from build123d import *

# Parameters (mm, degrees)
SKETCH1_W           = 12.5
SKETCH1_H           = 14
BOSS_EXTRUDE1_DEPTH = 5
CUT_EXTRUDE1_START  = -4.5
SKETCH3_W           = 0.63999998
SKETCH3_H           = 0.639999981
SKETCH3_W_2         = 0.639999981
CUT_EXTRUDE1_DEPTH  = 4.5
CHAMFER1_SIZE       = 0.5
CHAMFER1_SIZE2      = 0.181985117
SKETCH4_W           = 1.639999981
SKETCH4_H           = 1.639999981
SKETCH4_W_2         = 1.63999998
CUT_EXTRUDE2_DEPTH  = 6


with BuildPart() as part:
    # Sketch1 → Boss-Extrude1 (new body)
    with BuildSketch(Plane(origin=(0, 0, 0), x_dir=(1, 0, 0), z_dir=(0, 1, 0))):
        Rectangle(SKETCH1_W, SKETCH1_H)
    extrude(amount=BOSS_EXTRUDE1_DEPTH)

    # Sketch3 → Cut-Extrude1 (cut)
    with BuildSketch(Plane.XY.offset(7).offset(CUT_EXTRUDE1_START)):
        with Locations((-5.080001681, 1.230026097)):
            Rectangle(SKETCH3_W, SKETCH3_H)
        with Locations((-2.540001758, 1.230026097)):
            Rectangle(SKETCH3_W_2, SKETCH3_H)
        with Locations((-1.834e-06, 1.230026097)):
            Rectangle(SKETCH3_W_2, SKETCH3_H)
        with Locations((2.539998088, 1.230026097)):
            Rectangle(SKETCH3_W_2, SKETCH3_H)
        with Locations((5.079998012, 1.230026097)):
            Rectangle(SKETCH3_W_2, SKETCH3_H)
        with Locations((5.079998012, 3.770026019)):
            Rectangle(SKETCH3_W_2, SKETCH3_H)
        with Locations((2.539998088, 3.770026019)):
            Rectangle(SKETCH3_W_2, SKETCH3_H)
        with Locations((-1.834e-06, 3.770026019)):
            Rectangle(SKETCH3_W_2, SKETCH3_H)
        with Locations((-2.540001758, 3.770026019)):
            Rectangle(SKETCH3_W_2, SKETCH3_H)
        with Locations((-5.080001681, 3.770026019)):
            Rectangle(SKETCH3_W, SKETCH3_H)
    extrude(amount=CUT_EXTRUDE1_DEPTH, mode=Mode.SUBTRACT)

    # Chamfer1
    chamfer1_edges = [part.edges().sort_by_distance(p)[0] for p in [
        (4.759998021, 1.230026096, 7),
        (5.079998011, 0.910026106, 7),
        (2.539998088, 1.550026087, 7),
        (2.219998098, 1.230026096, 7),
        (2.539998088, 0.910026106, 7),
        (2.859998079, 1.230026096, 7),
        (0.319998156, 1.230026096, 7),
        (-1.835e-06, 1.550026087, 7),
        (-0.320001825, 1.230026096, 7),
        (-1.835e-06, 0.910026106, 7),
        (-2.220001767, 1.230026096, 7),
        (-2.540001758, 1.550026087, 7),
        (-2.860001748, 1.230026096, 7),
        (-2.540001758, 0.910026106, 7),
        (-5.080001681, 0.910026106, 7),
        (-4.760001691, 1.230026096, 7),
        (-5.080001681, 1.550026087, 7),
        (-5.400001671, 1.230026096, 7),
        (-5.080001681, 3.450026029, 7),
        (-4.760001691, 3.77002602, 7),
        (-5.080001681, 4.09002601, 7),
        (-5.400001671, 3.77002602, 7),
        (-2.540001758, 4.09002601, 7),
        (-2.860001748, 3.77002602, 7),
        (-2.540001758, 3.450026029, 7),
        (-2.220001767, 3.77002602, 7),
        (0.319998156, 3.77002602, 7),
        (-1.835e-06, 4.09002601, 7),
        (-0.320001825, 3.77002602, 7),
        (-1.835e-06, 3.450026029, 7),
        (2.859998079, 3.77002602, 7),
        (2.539998088, 4.09002601, 7),
        (2.219998098, 3.77002602, 7),
        (2.539998088, 3.450026029, 7),
        (5.079998011, 4.09002601, 7),
        (4.759998021, 3.77002602, 7),
        (5.079998011, 3.450026029, 7),
        (5.399998002, 3.77002602, 7),
        (5.399998002, 1.230026096, 7),
        (5.079998011, 1.550026087, 7),
    ]]
    chamfer1_side = [part.faces().sort_by_distance(p)[0] for p in [
        (1.29e-07, 2.499998172, 7),
    ]]
    chamfer(chamfer1_edges, length=CHAMFER1_SIZE, length2=CHAMFER1_SIZE2, reference=chamfer1_side[0])

    # Sketch4 → Cut-Extrude2 (cut)
    with BuildSketch(Plane(origin=(0, 0, -7), x_dir=(-1, 0, 0), z_dir=(0, 0, -1))):
        with Locations((-5.079998012, 1.230026097)):
            Rectangle(SKETCH4_W, SKETCH4_H)
        with Locations((-2.539998088, 1.230026097)):
            Rectangle(SKETCH4_W, SKETCH4_H)
        with Locations((1.835e-06, 1.230026097)):
            Rectangle(SKETCH4_W, SKETCH4_H)
        with Locations((2.540001758, 1.230026097)):
            Rectangle(SKETCH4_W, SKETCH4_H)
        with Locations((5.080001681, 1.230026097)):
            Rectangle(SKETCH4_W_2, SKETCH4_H)
        with Locations((5.080001681, 3.770026019)):
            Rectangle(SKETCH4_W_2, SKETCH4_H)
        with Locations((2.540001758, 3.770026019)):
            Rectangle(SKETCH4_W, SKETCH4_H)
        with Locations((1.835e-06, 3.770026019)):
            Rectangle(SKETCH4_W, SKETCH4_H)
        with Locations((-2.539998088, 3.770026019)):
            Rectangle(SKETCH4_W, SKETCH4_H)
        with Locations((-5.079998012, 3.770026019)):
            Rectangle(SKETCH4_W, SKETCH4_H)
    extrude(amount=-CUT_EXTRUDE2_DEPTH, mode=Mode.SUBTRACT)


solid = part.part
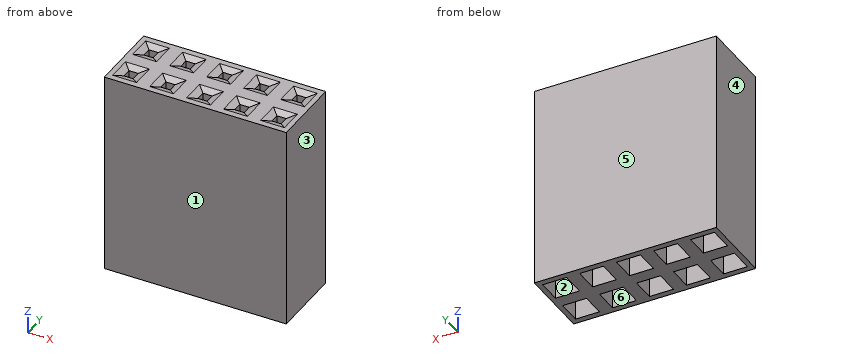
Read the model definition and answer for the solid it produces. Units are mm, in the model's axes. Face numbers are marked on the shaded views. A direction names the side the tool comes from. Give positions to 0.01 mm unless a question says otherwise; leave off trailing zeros. Loops run counter-clockwise (first coordinate to the right, second up) from the corner with the lowest first, then second, coordinate; pieces in that order, holes last. Notation, with made-up numbers: (22, 14) - (71, 14) arc R9 cw to (71, 21) - close; hole circle Ø5 at (46.25, 48.5). An arc over 180 degrees is marked (long way). Answer as CSV lines item,"result". Start each with the question number.
1) Straight lines are drawn through the part: L1, parallel to X at y = 1.6, z = -5.75; L2, parallel to Y at x = -2.5, z = -6; L3, parallel to Z at x = 3, y = 4.55. For each, find the intervals that lie inside material, in ascending order. Write a range as from..to.
2) Find section A-A (x = 2.5). Write down the section's boundary in (y, z), then the cut area to 3 significant figures.
3) Which of the six approach directions +Z, -Z, +X, -X, +Y, -Y give full straight-line access (tool end or side, diameter ignored) to the marked faces 1 and 2?
4) Find section B-B (z = -2). State how many separate pieces and enclosed holes the cut face has, then the cut area to 3 significant figures.
5) Determine the mould class of the marked faces 3, 4, 5 and 6 for opening direction X: released by +X, released by -X, zero draft, split by the parting line, or undercut.
6) Find section D-D (x = -0.5). Write down the section's boundary in (y, z).
7) Each of these flat-tipped pins is pushed along its axis until it touches: pin 1 Ø0.8 at (x, y) = (2.5, 3.5) entering from -Z; pin 2 Ø0.5 at (x, y) = (-5, 4) entering from +Z. Where does it stop, or does it pass through?
Findings below:
1,L1,"-6.25..-5.9, -4.26..-3.36, -1.72..-0.82, 0.82..1.72, 3.36..4.26, 5.9..6.25"
1,L2,"0..0.41, 2.05..2.95, 4.59..5"
1,L3,"-1..6.99"
2,outline,"(0, -7) - (0.41, -7) - (0.41, -1) - (2.05, -1) - (2.05, -7) - (2.95, -7) - (2.95, -1) - (4.59, -1) - (4.59, -7) - (5, -7) - (5, 7) - (4.59, 7) - (4.09, 6.82) - (4.09, 2.5) - (3.45, 2.5) - (3.45, 6.82) - (2.95, 7) - (2.05, 7) - (1.55, 6.82) - (1.55, 2.5) - (0.91, 2.5) - (0.91, 6.82) - (0.41, 7) - (0, 7) - close"
2,area,"44.4 mm^2"
3,face 1,"+Z, -Z, +X, -X, -Y"
3,face 2,"-Z"
4,separate pieces,"1"
4,enclosed holes,"10"
4,area,"35.6 mm^2"
5,face 3,"released by +X"
5,face 4,"released by -X"
5,face 5,"zero draft"
5,face 6,"undercut"
6,outline,"(0, -7) - (0.41, -7) - (0.41, -1) - (2.05, -1) - (2.05, -7) - (2.95, -7) - (2.95, -1) - (4.59, -1) - (4.59, -7) - (5, -7) - (5, 7) - (4.59, 7) - (4.27, 6.88) - (3.27, 6.88) - (2.95, 7) - (2.05, 7) - (1.73, 6.88) - (0.73, 6.88) - (0.41, 7) - (0, 7) - close"
7,pin 1,"z = -1"
7,pin 2,"z = 6.88"
